Read the model definition and answer for the solid it produces. Units are mm, in the model's axes. A direction names the side the tool comes from. Give positions to 0.01 mm unless a question says otherwise; leave off trailing zeros. Order: outer loops, then holes, each group sorted by start corner. A loop starts at its lowest first (then second) coordinate and runs counter-clockwise, first axis right, second up.
```python
from build123d import *

# Parameters (mm, degrees)
SKETCH_1_W          = 30
SKETCH_1_H          = 30
EXTRUDE_1_DEPTH     = 30
SKETCH_2_W          = 20
SKETCH_2_H          = 20.05
CUT_EXTRUDE_1_DEPTH = 20
CUT_EXTRUDE_2_DEPTH = 20
SKETCH_4_W          = 5
SKETCH_4_H          = 30
CUT_EXTRUDE_3_DEPTH = 55
SKETCH_5_W          = 15
SKETCH_5_H          = 4.975
EXTRUDE_2_DEPTH     = 120
EXTRUDE_3_DEPTH     = 60
SKETCH_7_R          = 3.1
CUT_EXTRUDE_4_DEPTH = 60
CUT_EXTRUDE_5_REACH = 155.704
SKETCH_8_W          = 20.1
SKETCH_8_H          = 20.15
EXTRUDE_4_DEPTH     = 1
SKETCH_10_W         = 26
SKETCH_10_H         = 15
CUT_EXTRUDE_6_DEPTH = 87


with BuildPart() as part:
    # 草图1 → 凸台-拉伸1 (new body)
    with BuildSketch(Plane(origin=(0, 0, 0), x_dir=(1, 0, 0), z_dir=(0, 1, 0))):
        Rectangle(SKETCH_1_W, SKETCH_1_H)
    extrude(amount=EXTRUDE_1_DEPTH)

    # 草图2 → 切除-拉伸1 (cut)
    with BuildSketch(Plane(origin=(15, 0, 0), x_dir=(0, 0, -1), z_dir=(1, 0, 0))):
        with Locations((5, 15)):
            Rectangle(SKETCH_2_W, SKETCH_2_H)
    extrude(amount=-CUT_EXTRUDE_1_DEPTH, mode=Mode.SUBTRACT)

    # 草图3 → 切除-拉伸2 (cut)
    with BuildSketch(Plane(origin=(-5, 0, 0), x_dir=(0, 0, -1), z_dir=(1, 0, 0))):
        with BuildLine():
            ThreePointArc((7.189292698, 17.194765929), (5, 18.1), (2.810707302, 17.194765929))
            Line((2.810707302, 17.194765929), (5, 15))
            Line((5, 15), (7.189292698, 17.194765929))
        make_face()
        with BuildLine():
            Line((5, 15), (2.810707302, 17.194765929))
            ThreePointArc((2.810707302, 17.194765929), (1.9, 15), (2.810707302, 12.805234071))
            Line((2.810707302, 12.805234071), (5, 15))
        make_face()
        with BuildLine():
            Line((7.189292698, 17.194765929), (5, 15))
            Line((5, 15), (7.189292698, 12.805234071))
            ThreePointArc((7.189292698, 12.805234071), (7.86328547, 13.81189381), (8.1, 15))
            ThreePointArc((8.1, 15), (7.86328547, 16.18810619), (7.189292698, 17.194765929))
        make_face()
        with BuildLine():
            Line((7.189292698, 12.805234071), (5, 15))
            Line((5, 15), (2.810707302, 12.805234071))
            ThreePointArc((2.810707302, 12.805234071), (5, 11.9), (7.189292698, 12.805234071))
        make_face()
    extrude(amount=-CUT_EXTRUDE_2_DEPTH, mode=Mode.SUBTRACT)

    # 草图4 → 切除-拉伸3 (cut)
    with BuildSketch(Plane.XZ):
        with Locations((-12.5, 0)):
            Rectangle(SKETCH_4_W, SKETCH_4_H)
    extrude(amount=-CUT_EXTRUDE_3_DEPTH, mode=Mode.SUBTRACT)

    # 草图5 → 凸台-拉伸2 (add)
    with BuildSketch(Plane(origin=(0, 0, -15), x_dir=(-1, 0, 0), z_dir=(0, 0, -1))):
        with Locations((-7.5, 27.5125)):
            Rectangle(SKETCH_5_W, SKETCH_5_H)
        with Locations((-7.5, 2.4875)):
            Rectangle(SKETCH_5_W, SKETCH_5_H)
    extrude(amount=EXTRUDE_2_DEPTH)

    # 草图6 → 凸台-拉伸3 (add)
    with BuildSketch(Plane(origin=(0, 0, -135), x_dir=(-1, 0, 0), z_dir=(0, 0, -1))):
        Polygon((5, 4.975), (0, 4.975), (0, 0), (10, 0), (10, 30), (0, 30), (0, 25.025), (5, 25.025), align=None)
    extrude(amount=-EXTRUDE_3_DEPTH)

    # 草图7 → 切除-拉伸4 (cut)
    with BuildSketch(Plane.ZY.offset(10)):
        with Locations((-105, 15)):
            Circle(SKETCH_7_R)
        with Locations((-85, 15)):
            Circle(SKETCH_7_R)
    extrude(amount=-CUT_EXTRUDE_4_DEPTH, mode=Mode.SUBTRACT)

    # 切除-拉伸5: up to this face of the body (flat: up to its plane)
    cut_extrude_5_end = Plane(part.part.faces().sort_by_distance((5, 15, 5))[0])
    # 草图8 → 切除-拉伸5 (cut, up to the picked face)
    with BuildSketch(Plane(origin=(0, 0, -135), x_dir=(-1, 0, 0), z_dir=(0, 0, -1)), mode=Mode.PRIVATE) as cut_extrude_5_sk1:
        with Locations((-5, 15)):
            Rectangle(SKETCH_8_W, SKETCH_8_H)
    cut_extrude_5_tool1 = split(extrude(cut_extrude_5_sk1.sketch, amount=-CUT_EXTRUDE_5_REACH, mode=Mode.PRIVATE), bisect_by=cut_extrude_5_end, keep=Keep.BOTH, mode=Mode.PRIVATE)
    add(cut_extrude_5_tool1.solids().sort_by(Axis((5, 15, -135), (0, 0, 1)))[0], mode=Mode.SUBTRACT)

    # 草图9 → 凸台-拉伸4 (add)
    with BuildSketch(Plane(origin=(15, 0, 0), x_dir=(0, 0, -1), z_dir=(1, 0, 0))):
        Polygon((135, 4.925), (-5, 4.925), (-5, 25.075), (135, 25.075), (135, 30), (-15, 30), (-15, 0), (135, 0), align=None)
    extrude(amount=EXTRUDE_4_DEPTH)

    # 草图10 → 切除-拉伸6 (cut)
    with BuildSketch(Plane.XZ):
        with Locations((3, -127.5)):
            Rectangle(SKETCH_10_W, SKETCH_10_H)
    extrude(amount=-CUT_EXTRUDE_6_DEPTH, mode=Mode.SUBTRACT)


solid = part.part
```
1) The part is cut by section C-C on x = 13.25. Determine the outline of the cut face in (y, z) (3 decimals).
Final values:
outline: (0, -120) - (4.925, -120) - (4.925, 5) - (25.075, 5) - (25.075, -120) - (30, -120) - (30, 15) - (0, 15) - close
2) The part is cut by section B-B on y = 10.75. Determine the outline of the cut face in (x, z).
Final values:
outline: (-10, -120) - (-5.05, -120) - (-5.05, -75) - (-10, -75) - close; (-10, -15) - (-5.05, -15) - (-5.05, 5) - (16, 5) - (16, 15) - (-10, 15) - close
3) The part is cut by section D-D on z = -79. Determine the outline of the cut face in (x, y) (3 decimals), and give its area (3 significant figures).
Final values:
outline: (-10, 0) - (16, 0) - (16, 4.925) - (-5.05, 4.925) - (-5.05, 25.075) - (16, 25.075) - (16, 30) - (-10, 30) - close
area: 356 mm2
4) The part is cut by section A-A on z = -105. Determine the outline of the cut face in (x, y) (3 decimals), and give its area (3 significant figures).
Final values:
outline: (-10, 0) - (16, 0) - (16, 4.925) - (-5.05, 4.925) - (-5.05, 11.9) - (-10, 11.9) - close; (-10, 18.1) - (-5.05, 18.1) - (-5.05, 25.075) - (16, 25.075) - (16, 30) - (-10, 30) - close
area: 325 mm2
5) Consider L1, parallel to Y at x = 4.25, z = -98.5 (3 decimals); L2, parallel to X at y = 24, z = -89.5; L3, parallel to Z at x = 2.25, y = 12.25. Determine where each line is inside the solid, lowest interval first.
Final values:
L1: y = 0 to 4.925, 25.075 to 30
L2: x = -10 to -5.05
L3: z = 5 to 15
6) Given pin 1 (4 mm diameter, centred on y = 28, z = -52, fed in from -X); pin 2 (4 mm diameter, centred on y = 22.5, z = -105, fed in from +X), each flat-ended and moving along its own axis, determine where each tip first touches the part or whether it passes through.
Final values:
pin 1: stops at x = 0
pin 2: stops at x = -5.05
7) A tool of negligible diameter and unlimited length cuts with its end or side. For faces 4 (the face through (0, 28, -45)), 5 (the face through (3, 15, 15)), 6 (the face through (-5.05, 15, -98)), from which of +Z, -Z, +X, -X, +Y, -Y can it reach the whole face along a straight path? Write none if from no direction.
Final values:
face 4: -X, +Y, -Y
face 5: +Z, +X, -X, +Y, -Y
face 6: -Z, +X
8) For a pull along Z with two mould halves and no side action, classify faces 1 (the face through (0, 2, -45)), 2 (the face through (-6, 11, -120)), 3 (the face through (6, 0, -52)) as released by +Z, released by -Z, zero draft, split by the parting line, or undercut.
Final values:
face 1: undercut
face 2: released by -Z
face 3: zero draft
